```python
from build123d import *

# Parameters (mm, degrees)
F0_R     = 1.75
F0_R_2   = 3.25
F1_DEPTH = 2
F3_DEPTH = 25


# Not quite as in the source:
# - a feature names something its author has since deleted; it is built from what else it names


with BuildPart() as f1:
    # F0 (on Top) → F1 (new body)
    with BuildSketch(Plane.XY):
        with BuildLine():
            ThreePointArc((-12.5717246149, 50.2695334528), (-16.1191217808, 44.4802479149), (-20.6904345264, 39.4599935911))
            ThreePointArc((-20.6904345264, 39.4599935911), (-21.8414434806, 37.6150390062), (-21.8571428571, 35.4405430733))
            ThreePointArc((-21.8571428571, 35.4405430733), (-20.4663771338, 28.6163953155), (-20, 21.6676030258))
            Line((-20, 21.6676030258), (-20, -10.6856030045))
            ThreePointArc((-20, -10.6856030045), (-19.7308995433, -13.9554047127), (-18.9308396789, -17.1372159077))
            Line((-18.9308396789, -17.1372159077), (-17.0470641697, -22.6647409918))
            ThreePointArc((-17.0470641697, -22.6647409918), (-16.9162578432, -26.0979642803), (-18.6905264293, -29.0400899451))
            ThreePointArc((-18.6905264293, -29.0400899451), (-19.7861679358, -33.2903225806), (-16.3230484377, -35.9869336221))
            ThreePointArc((-16.3230484377, -35.9869336221), (-13.1213600073, -37.2332576723), (-11.1283691906, -40.0318501842))
            Line((-11.1283691906, -40.0318501842), (-10.837240035, -40.8861046865))
            ThreePointArc((-10.837240035, -40.8861046865), (-9.4747581102, -42.9666501557), (-7.2784782144, -44.1334325108))
            ThreePointArc((-7.2784782144, -44.1334325108), (-3.6649414842, -44.7825957956), (0, -45))
            ThreePointArc((0, -45), (3.6649414842, -44.7825957956), (7.2784782144, -44.1334325108))
            ThreePointArc((7.2784782144, -44.1334325108), (9.4747581102, -42.9666501557), (10.837240035, -40.8861046865))
            Line((10.837240035, -40.8861046865), (11.1283691906, -40.0318501842))
            ThreePointArc((11.1283691906, -40.0318501842), (13.1213600073, -37.2332576723), (16.3230484377, -35.9869336221))
            ThreePointArc((16.3230484377, -35.9869336221), (19.7861679358, -33.2903225806), (18.6905264293, -29.0400899451))
            ThreePointArc((18.6905264293, -29.0400899451), (16.9162578432, -26.0979642803), (17.0470641697, -22.6647409918))
            Line((17.0470641697, -22.6647409918), (18.9308396789, -17.1372159077))
            ThreePointArc((18.9308396789, -17.1372159077), (19.7308995433, -13.9554047127), (20, -10.6856030045))
            Line((20, -10.6856030045), (20, 21.6676030258))
            ThreePointArc((20, 21.6676030258), (20.4663771338, 28.6163953155), (21.8571428571, 35.4405430733))
            ThreePointArc((21.8571428571, 35.4405430733), (21.8414434806, 37.6150390062), (20.6904345264, 39.4599935911))
            ThreePointArc((20.6904345264, 39.4599935911), (16.1191217808, 44.4802479149), (12.5717246149, 50.2695334528))
            ThreePointArc((12.5717246149, 50.2695334528), (10.6050430884, 51.2048486848), (9.25, 49.5))
            Line((9.25, 49.5), (9.25, 38))
            ThreePointArc((9.25, 38), (0, 28.75), (-9.25, 38))
            Line((-9.25, 38), (-9.25, 49.5))
            ThreePointArc((-9.25, 49.5), (-10.6050430884, 51.2048486848), (-12.5717246149, 50.2695334528))
        make_face()
        with Locations((-16, -32)):
            Circle(F0_R, mode=Mode.SUBTRACT)
        with BuildLine():
            Line((-17.5, -1.5), (-17.5, 1.5))
            ThreePointArc((-17.5, 1.5), (-16.5, 2.5), (-15.5, 1.5))
            Line((-15.5, 1.5), (-15.5, -1.5))
            ThreePointArc((-15.5, -1.5), (-16.5, -2.5), (-17.5, -1.5))
        make_face(mode=Mode.SUBTRACT)
        with BuildLine():
            Line((-13, -7), (-13, 7))
            ThreePointArc((-13, 7), (-12, 8), (-11, 7))
            Line((-11, 7), (-11, -7))
            ThreePointArc((-11, -7), (-12, -8), (-13, -7))
        make_face(mode=Mode.SUBTRACT)
        with Locations((0, -38)):
            Circle(F0_R_2, mode=Mode.SUBTRACT)
        with Locations((0, -26)):
            Circle(F0_R_2, mode=Mode.SUBTRACT)
        with Locations((16, -32)):
            Circle(F0_R, mode=Mode.SUBTRACT)
        with BuildLine():
            Line((10.5, -14.5), (-10.5, -14.5))
            ThreePointArc((-10.5, -14.5), (-11.75, -13.25), (-10.5, -12))
            Line((-10.5, -12), (10.5, -12))
            ThreePointArc((10.5, -12), (11.75, -13.25), (10.5, -14.5))
        make_face(mode=Mode.SUBTRACT)
        with BuildLine():
            Line((11, -7), (11, 7))
            ThreePointArc((11, 7), (12, 8), (13, 7))
            Line((13, 7), (13, -7))
            ThreePointArc((13, -7), (12, -8), (11, -7))
        make_face(mode=Mode.SUBTRACT)
        with BuildLine():
            Line((15.5, -1.5), (15.5, 1.5))
            ThreePointArc((15.5, 1.5), (16.5, 2.5), (17.5, 1.5))
            Line((17.5, 1.5), (17.5, -1.5))
            ThreePointArc((17.5, -1.5), (16.5, -2.5), (15.5, -1.5))
        make_face(mode=Mode.SUBTRACT)
        with Locations((-18, 36.5)):
            Circle(F0_R, mode=Mode.SUBTRACT)
        with BuildLine():
            Line((10.5, 12), (-10.5, 12))
            ThreePointArc((-10.5, 12), (-11.75, 13.25), (-10.5, 14.5))
            Line((-10.5, 14.5), (10.5, 14.5))
            ThreePointArc((10.5, 14.5), (11.75, 13.25), (10.5, 12))
        make_face(mode=Mode.SUBTRACT)
        with Locations((18, 36.5)):
            Circle(F0_R, mode=Mode.SUBTRACT)
    extrude(amount=F1_DEPTH)

    # F2 (on face) → F3 (cut)
    with BuildSketch(Plane.XY.offset(2)):
        with BuildLine():
            Line((1.0502525317, 8), (-1.0502525317, 8))
            ThreePointArc((-1.0502525317, 8), (-2.8980115967, 6.7653668647), (-2.4644660941, 4.5857864376))
            Line((-2.4644660941, 4.5857864376), (-1.4142135624, 3.5355339059))
            ThreePointArc((-1.4142135624, 3.5355339059), (0, 2.9497474683), (1.4142135624, 3.5355339059))
            Line((1.4142135624, 3.5355339059), (2.4644660941, 4.5857864376))
            ThreePointArc((2.4644660941, 4.5857864376), (2.8980115967, 6.7653668647), (1.0502525317, 8))
        make_face()
        with BuildLine():
            ThreePointArc((-2.4644660941, -4.5857864376), (-2.8980115967, -6.7653668647), (-1.0502525317, -8))
            Line((-1.0502525317, -8), (1.0502525317, -8))
            ThreePointArc((1.0502525317, -8), (2.8980115967, -6.7653668647), (2.4644660941, -4.5857864376))
            Line((2.4644660941, -4.5857864376), (1.4142135624, -3.5355339059))
            ThreePointArc((1.4142135624, -3.5355339059), (0, -2.9497474683), (-1.4142135624, -3.5355339059))
            Line((-1.4142135624, -3.5355339059), (-2.4644660941, -4.5857864376))
        make_face()
        with BuildLine():
            ThreePointArc((-4.5857864376, 2.4644660941), (-6.7653668647, 2.8980115967), (-8, 1.0502525317))
            Line((-8, 1.0502525317), (-8, -1.0502525317))
            ThreePointArc((-8, -1.0502525317), (-6.7653668647, -2.8980115967), (-4.5857864376, -2.4644660941))
            Line((-4.5857864376, -2.4644660941), (-3.5355339059, -1.4142135624))
            ThreePointArc((-3.5355339059, -1.4142135624), (-2.9497474683, 0), (-3.5355339059, 1.4142135624))
            Line((-3.5355339059, 1.4142135624), (-4.5857864376, 2.4644660941))
        make_face()
        with BuildLine():
            Line((8, -1.0502525317), (8, 1.0502525317))
            ThreePointArc((8, 1.0502525317), (6.7653668647, 2.8980115967), (4.5857864376, 2.4644660941))
            Line((4.5857864376, 2.4644660941), (3.5355339059, 1.4142135624))
            ThreePointArc((3.5355339059, 1.4142135624), (2.9497474683, 0), (3.5355339059, -1.4142135624))
            Line((3.5355339059, -1.4142135624), (4.5857864376, -2.4644660941))
            ThreePointArc((4.5857864376, -2.4644660941), (6.7653668647, -2.8980115967), (8, -1.0502525317))
        make_face()
        with BuildLine():
            ThreePointArc((-5.0763219385, 20.5680916489), (-5.7238553417, 18.3428026544), (-3.8349160497, 17))
            Line((-3.8349160497, 17), (3.8349160497, 17))
            ThreePointArc((3.8349160497, 17), (5.7238553417, 18.3428026544), (5.0763219385, 20.5680916489))
            Line((5.0763219385, 20.5680916489), (1.2414058887, 23.604066855))
            ThreePointArc((1.2414058887, 23.604066855), (0, 24.035975206), (-1.2414058887, 23.604066855))
            Line((-1.2414058887, 23.604066855), (-5.0763219385, 20.5680916489))
        make_face()
        with BuildLine():
            ThreePointArc((-8.5714285714, 29.6017494533), (-10.755928946, 30.0536812284), (-12, 28.2020410289))
            Line((-12, 28.2020410289), (-12, 23.0473581273))
            ThreePointArc((-12, 23.0473581273), (-10.870973083, 21.246967645), (-8.7585941113, 21.4792664784))
            Line((-8.7585941113, 21.4792664784), (-5.4230382746, 24.1199148491))
            ThreePointArc((-5.4230382746, 24.1199148491), (-4.6719651901, 25.8612910654), (-5.7123807114, 27.4468627126))
            ThreePointArc((-5.7123807114, 27.4468627126), (-7.2227201333, 28.4170821836), (-8.5714285714, 29.6017494533))
        make_face()
        with BuildLine():
            Line((12, 23.0473581273), (12, 28.2020410289))
            ThreePointArc((12, 28.2020410289), (10.755928946, 30.0536812284), (8.5714285714, 29.6017494533))
            ThreePointArc((8.5714285714, 29.6017494533), (7.2227201333, 28.4170821836), (5.7123807114, 27.4468627126))
            ThreePointArc((5.7123807114, 27.4468627126), (4.6719651901, 25.8612910654), (5.4230382746, 24.1199148491))
            Line((5.4230382746, 24.1199148491), (8.7585941113, 21.4792664784))
            ThreePointArc((8.7585941113, 21.4792664784), (10.870973083, 21.246967645), (12, 23.0473581273))
        make_face()
    extrude(amount=-F3_DEPTH, mode=Mode.SUBTRACT)


solid = f1.part
```
Work out the finished part from the listing and answer in its coordinate system (mm). A direction names the side the tool comes from. Give positions to 0.01 mm unless a question says otherwise; leave off trailing zeros. Loops run counter-clockwise (first coordinate to the right, second up) from the corner with the lowest first, then second, coordinate; pieces in that order, holes last. Notation, with made-up numbers: (8, 74.5) - (14, 74.5) arc R31 ccw to (14, 102.5) - close; hole circle Ø11 at (14, 50.5). An arc over 180 degrees is marked (long way). One line per question, with ' | ' between items.
(1) The part is cut by section B-B (z = 1.05). Count the separate pieces of the cut face and the enclosed holes in it, then the cut area to 3 significant figures.
Recorded:
separate pieces: 1 | enclosed holes: 19 | area: 2,610 mm²
(2) The part is cut by section C-C (y = -13.25). Write down the section's boundary in (x, z), then the cut area to 3 significant figures.
Recorded:
outline: (-19.83, 0) - (-11.75, 0) - (-11.75, 2) - (-19.83, 2) - close; (11.75, 0) - (19.83, 0) - (19.83, 2) - (11.75, 2) - close | area: 32.3 mm²
(3) The part is cut by section A-A (y = 43). Write down the section's boundary in (x, z).
Recorded:
outline: (-17.29, 0) - (-9.25, 0) - (-9.25, 2) - (-17.29, 2) - close; (9.25, 0) - (17.29, 0) - (17.29, 2) - (9.25, 2) - close
(4) Straight lines are drawn through the part: probe 1 along Y at (x, z) = (-6.5, 0.65); probe 2 along X at (y, z) = (38, 0.85); probe 3 along X at (y, z) = (25, 1.15). For each, find the intervals that lie inside material, in ascending order.
Recorded:
probe 1: y = -44.31 to -14.5, -12 to -2.99, 2.99 to 12, 14.5 to 23.27, 27.91 to 31.42 | probe 2: x = -21.71 to -18.9, -17.1 to -9.25, 9.25 to 17.1, 18.9 to 21.71 | probe 3: x = -20.11 to -12, -4.79 to 4.79, 12 to 20.11
(5) A tool of negligible diameter and unlimited length cuts with its end or side. For faces 5 (the face through (-16.904, -26.051, 0.986)), 6 (the face through (16.5, 2.5, 1)), 7 (the face through (17.976, -19.94, 0.986)), 8 (the face through (-20, 6, 1)), from which of +Z, -Z, +X, -X, +Y, -Y can it reach the whole face along a straight path? Write none if from no direction.
Recorded:
face 5: +Z, -Z, -X | face 6: +Z, -Z | face 7: +Z, -Z, +X | face 8: +Z, -Z, -X, -Y
(6) The mould has two halves that part along X. Classify faces 1 (the face through (-13.16, -37.203, 0.986)), 2 (the face through (7.2, 28.4, 1)), 3 (the face through (16.18, 44.4, 0.99)), 4 (the face through (2.91, 6.735, 1.014)): +X half, -X half, draft (parallel to the pull), parting line (faces both ways), or undercut.
Recorded:
face 1: -X half | face 2: undercut | face 3: +X half | face 4: undercut
(7) Each of these flat-tipped pins is pushed along its axis until it touches: pin 1 Ø3 at (x, y) = (-4, 5) entering from -Z; pin 2 Ø0.6 at (x, z) = (1, 1) entering from +Y; pin 3 Ø2 at (x, y) = (-16, -32) entering from -Z; pin 4 Ø1 at (x, z) = (15.5, 0.5) entering from +Y. Where does it stop, or does it pass through?
Recorded:
pin 1: stops at z = 0 | pin 2: stops at y = 28.84 | pin 3: passes through | pin 4: stops at y = 46.06
